Can you work these out from the drawing? Everything is in mm from the part's minimum corner. A direction names the side the tool comes from. Give positions to 0.01 mm unless a question says otherwise; leave off trailing zeros. Write each loop counter-clockwise with the first axis right and the second up, starting at its lowest first coordinate (ties: lowest second). Pieces come first, ordered by that corner, then holes. Notation, with made-up numbers: (13.5, 49.25) - (47.5, 49.25) arc R25 ccw to (47.5, 88.25) - close; hole circle Ø1 at (-29.5, 28.5). An arc over 180 degrees is marked (long way). Write each question's results on one line, items separated by ' | '. Start each with the question number.
Item 1: Will these pins go through, and if not, where does the flat tip stop? P1, Ø1.5, axis at y = 30, z = 27, coming from the +X side; P2, Ø24, axis at y = 16.5, z = 27.5, coming from the -X side.
Item 2: Please list where these lines run through material, in increasing order: line 1 along Z through (x, y) = (50, 14.5); line 2 along X through (y, z) = (39, 39.5) (1 decimal); line 3 along X through (y, z) = (42.5, 12).
Item 3: We'd pull the mould along X, two halves only. Please class the marked faces 4, 5 and 6: +X half, -X half, draft (parallel to the pull), parting line (faces both ways), or undercut.
Item 4: Which directions (+Z, -Z, +X, -X, +Y, -Y) give clear straight access to the entire face, cutting with the end or side of a thin tool? Please do the marked faces 1, 2 and 3.
Item 5: Suppose I cut it at D-D on z = 46.5. List the corners of the cut face in (x, y) for me, then the cut area to 3 significant figures.
Item 6: Suppose I cut it at A-A on x = 50. List the corners of the cut face in (y, z) for me.
Item 7: Suppose I cut it at C-C on z = 30. List the corners of the cut face in (x, y) for me.
Item 8: Suppose I cut it at B-B on y = 11. List the corners of the cut face in (x, z) for me, then the cut area to 3 significant figures.
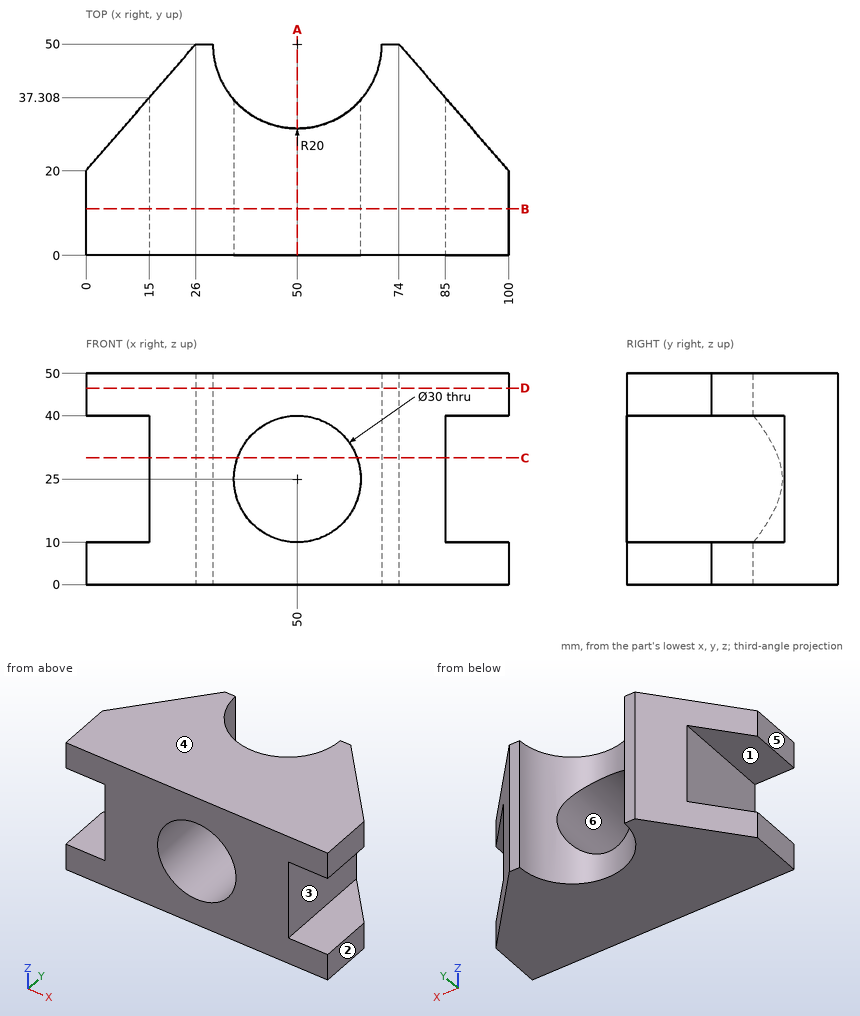
Checked values:
1) P1: stops at x = 85 | P2: stops at x = 15
2) line 1: z = 0 to 10, 40 to 50 | line 2: x = 16.5 to 33.3, 66.7 to 83.5 | line 3: x = 19.5 to 31.46, 68.54 to 80.5
3) face 4: draft | face 5: -X half | face 6: undercut
4) face 1: -X, +Y, -Y | face 2: +Z, -Z, +X, +Y, -Y | face 3: +X, +Y, -Y
5) outline: (0, 0) - (100, 0) - (100, 20) - (74, 50) - (70, 50) arc R20 cw to (30, 50) - (26, 50) - (0, 20) - close | area: 3,590 mm^2
6) outline: (0, 0) - (30, 0) - (30, 10) - (0, 10) - close; (0, 40) - (30, 40) - (30, 50) - (0, 50) - close
7) outline: (15, 0) - (35.86, 0) - (35.86, 35.86) arc R20 cw to (30, 50) - (26, 50) - (15, 37.31) - close; (64.14, 0) - (85, 0) - (85, 37.31) - (74, 50) - (70, 50) arc R20 cw to (64.14, 35.86) - close
8) outline: (0, 0) - (100, 0) - (100, 10) - (85, 10) - (85, 40) - (100, 40) - (100, 50) - (0, 50) - (0, 40) - (15, 40) - (15, 10) - (0, 10) - close; hole circle Ø30 at (50, 25) | area: 3,390 mm^2
